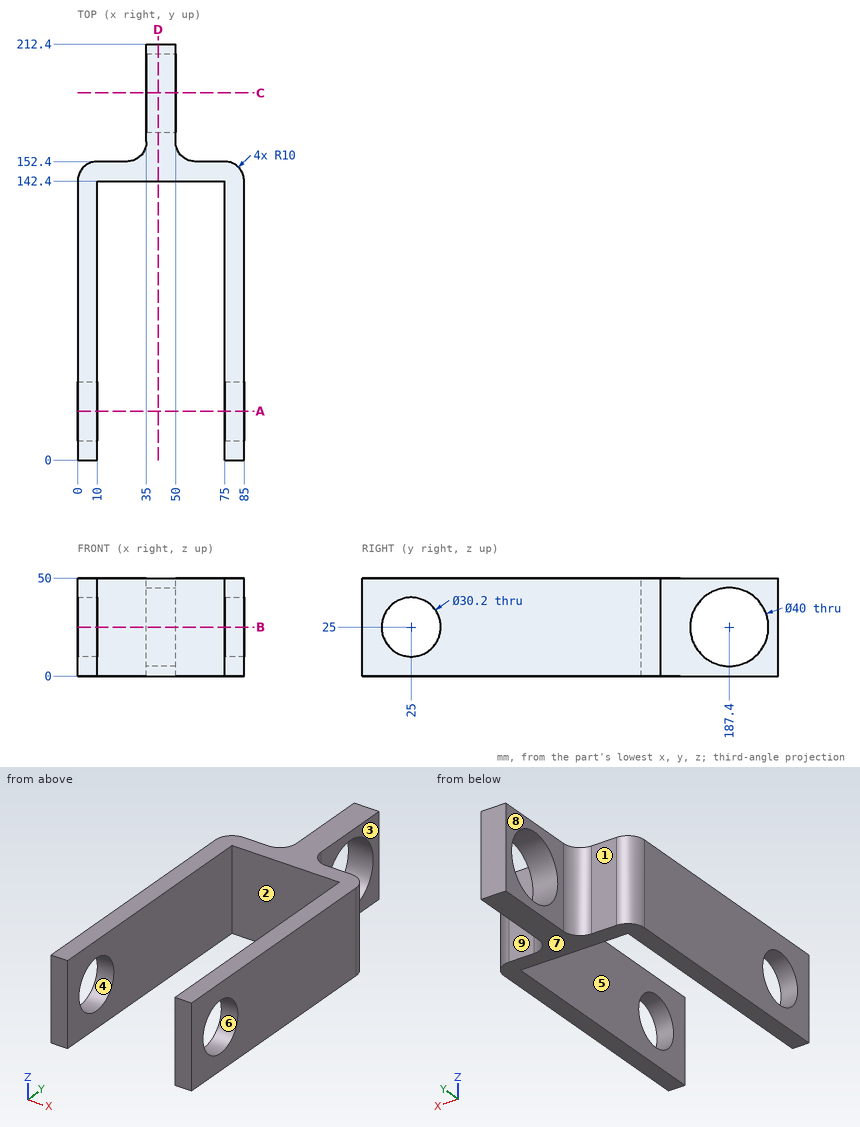
Answer from the drawing. Dimensions are ordinates in mm from the lowest x, y and z of the part. A direction names the side the tool comes from. Give positions to 0.01 mm unless a question says otherwise; leave off trailing zeros. Order: outer loops, then holes, each group sorted by start corner. A loop starts at its lowest first (then second) coordinate and runs counter-clockwise, first axis right, second up. Notation, with made-up numbers: (77.25, 46) -> (133.25, 46) arc R25 cw to (133.25, 80) -> close; hole circle Ø10 at (53, -11). An arc over 180 degrees is marked (long way). Answer as a JSON object with one key per item and string values. Group by question number.
1. The mould has two halves that part along Y. Classify the marked faces 1, 2, 3 and 4: released by +Y, released by -Y, zero draft, split by the parting line, or undercut.
2. Section C-C on y = 187.4 is taken. Determine the outline of the cut face in (x, z).
3. Flat-ended cylindrical pins translate along their axes: pin 1 Ø4 at (x, z) = (10, 30) entering from +Y; pin 2 Ø2 at (x, z) = (59.5, 9) entering from +Y; pin 3 Ø15 at (y, z) = (182, 18) entering from +X. Find the tip coordinate at first contact, or state that the pin passes through.
4. Section D-D on x = 41 is taken. Determine the outline of the cut face in (y, z), plus the area to 3 significant figures.
5. Consider line 1 along X through (y, z) = (82, 42.5); line 2 along Y through (x, z) = (44, 25); line 3 along X through (y, z) = (190, 3.5). Determine where each line is inside the solid, lowest interval first. Write a range as [from, to].
6. A tool of negligible diameter and unlimited length cuts with its end or side. For the marked faces 5, 6, 7, 8 and 9, from which of +Z, -Z, +X, -X, +Y, -Y can it reach the whole face along a straight path? Write none if from no direction.
7. Section B-B on z = 25 is taken. Determine the outline of the cut face in (x, y), plus the area to 3 significant figures.
8. Section A-A on y = 25 is taken. Determine the outline of the cut face in (x, z), plus the area to 3 significant figures.
Result sheet:
{
 "1": {"face 1": "released by +Y", "face 2": "released by -Y", "face 3": "zero draft", "face 4": "undercut"},
 "2": {"outline": "(35, 0) -> (50, 0) -> (50, 5) -> (35, 5) -> close; (35, 45) -> (50, 45) -> (50, 50) -> (35, 50) -> close"},
 "3": {"pin 1": "stops at y = 152.4", "pin 2": "stops at y = 152.51", "pin 3": "passes through"},
 "4": {"outline": "(142.4, 0) -> (212.4, 0) -> (212.4, 50) -> (142.4, 50) -> close; hole circle Ø40 at (187.4, 25)", "area": "2,240 mm^2"},
 "5": {"line 1": "x = [0, 10], [75, 85]", "line 2": "y = [142.4, 167.4], [207.4, 212.4]", "line 3": "x = [35, 50]"},
 "6": {"face 5": "+Z, -Z, -Y", "face 6": "+X, -X", "face 7": "-Z, +X, -X, +Y, -Y", "face 8": "+Z, -Z, -X, +Y", "face 9": "+Z, -Z, +X, +Y"},
 "7": {"outline": "(0, 0) -> (10, 0) -> (10, 9.9) -> (0, 9.9) -> close; (0, 40.1) -> (10, 40.1) -> (10, 142.4) -> (75, 142.4) -> (75, 40.1) -> (85, 40.1) -> (85, 142.4) arc R10 ccw to (75, 152.4) -> (60, 152.4) arc R10 cw to (50, 162.4) -> (50, 167.4) -> (35, 167.4) -> (35, 162.4) arc R10 cw to (25, 152.4) -> (10, 152.4) arc R10 ccw to (0, 142.4) -> close; (35, 207.4) -> (50, 207.4) -> (50, 212.4) -> (35, 212.4) -> close; (75, 0) -> (85, 0) -> (85, 9.9) -> (75, 9.9) -> close", "area": "3,390 mm^2"},
 "8": {"outline": "(0, 0) -> (10, 0) -> (10, 9.9) -> (0, 9.9) -> close; (0, 40.1) -> (10, 40.1) -> (10, 50) -> (0, 50) -> close; (75, 0) -> (85, 0) -> (85, 9.9) -> (75, 9.9) -> close; (75, 40.1) -> (85, 40.1) -> (85, 50) -> (75, 50) -> close", "area": "396 mm^2"}
}
